Input: part model. Units: mm. Frame: model coordinates. A direction names the side the tool comes from. Coordinates: 2 decimals unless noted, no trailing zeros. Use a Markdown table: item, result. Add a question column.
Autodesk Inventor part; units mm, degrees
ref_plane "YZ Plane" through (0, 0, 0) normal (1, 0, 0) x (0, 1, 0)
ref_plane "XZ Plane" through (0, 0, 0) normal (0, 1, 0) x (-1, 0, 0)
ref_plane "XY Plane" through (0, 0, 0) normal (0, 0, 1) x (1, 0, 0)
sketch "Sketch1" plane through (0, 0, 0) normal (0, 1, 0) x (-1, 0, 0)
  line L0 (0, 0) -> (-40, 0)
  line L1 (-40, 0) -> (-40, -50)
  line L2 (-40, -50) -> (0, -50)
  line L3 (0, -50) -> (0, 0)
  dimension "d0" = 40
  dimension "d1" = 50
extrude "Extrusion1" add sketch "Sketch1" along normal blind 100
move faces "Move1" translate (0, 0, -13) faces at (13.3333, 33.3333, 0)
sketch "Sketch2" plane through (0, 0, -13) normal (0, 0, 1) x (1, 0, 0)
  line L0 (0, 0) -> (40, 0)
  line L1 (40, 0) -> (40, 100)
  line L2 (0, 100) -> (40, 100)
  line L3 (0, 0) -> (0, 100)
  line L4 (39, 99) -> (39, 1)
  line L5 (39, 1) -> (1, 1)
  line L6 (1, 1) -> (1, 99)
  line L7 (1, 99) -> (39, 99)
  dimension "d7" = 1
extrude "Extrusion2" add sketch "Sketch2" along normal blind 2 contours L4 L5 L6 L7
sketch "Sketch3" plane through (0, 0, -11) normal (0, 0, 1) x (1, 0, 0)
  line L0 (0, 100) -> (40, 100)
  line L1 (0, 0) -> (0, 100)
  line L2 (40, 0) -> (40, 100)
  line L3 (0, 0) -> (40, 0)
extrude "Extrusion3" add sketch "Sketch3" along normal blind 12
move faces "Move2" translate (3, 0, 0) faces at (40, 66.6667, -37.6667) (39, 33.6667, -12.3333) (40, 33.3333, -7)
move faces "Move3" translate (0, -3, 0) faces at (28.6667, 100, -25.3333) (14.6667, 99, -11.6667) (14.3333, 100, -3)
sketch "Sketch4" plane through (0, 0, 1) normal (0, 0, 1) x (1, 0, 0)
  line L0 (0, 97) -> (0, 0)
  line L1 (0, 0) -> (43, 0)
  line L2 (43, 0) -> (43, 97)
  line L3 (43, 97) -> (0, 97)
  line L4 (1, 96) -> (1, 1)
  line L5 (1, 1) -> (42, 1)
  line L6 (42, 1) -> (42, 96)
  line L7 (42, 96) -> (1, 96)
  line L8 (1, 96) -> (42, 96)
  line L9 (1, 96) -> (11, 96)
  line L10 (11, 96) -> (11, 86)
  line L11 (11, 86) -> (1, 86)
  line L12 (1, 86) -> (1, 96)
  line L13 (42, 96) -> (32, 96)
  line L14 (32, 96) -> (32, 86)
  line L15 (32, 86) -> (42, 86)
  line L16 (42, 86) -> (42, 96)
  dimension "d18" = 1
  dimension "d19" = 10
  dimension "d20" = 10
  dimension "d21" = 10
  dimension "d22" = 10
extrude "Extrusion4" cut sketch "Sketch4" against normal blind 0.5 contours L7 L10 L11 L4 | L7 L6 L15 L14
ref_plane "Work Plane1" through (0, 48.5, 0) normal (0, -1, 0) x (1, 0, 0)
equation "\"d22\" = d20"
properties part number "1.4AH SLAB"
1) Contact query for flat-ended pins moving along their axis: P1, Ø3, axis at x = 35, y = 90, coming from the +Z side; P2, Ø8, axis at x = 7.5, y = 90, coming from the +Z side; P3, Ø0.6, axis at x = 30.5, z = -12, coming from the +Y side; P4, Ø0.6, axis at x = 20, z = -11.5, coming from the -Y side. Output: stop coordinate, or through.
2) Material intervals for L1, parallel to Y at x = 34.5, z = -12, sorted ascending.
3) Pull-direction query (Z, two-part tool) for faces 1 (the flat face through (6, 91, 0.5)), 2 (the flat face through (22, 0, -31)), 3 (the flat face through (1, 48, -12)); classes: pulls with the +Z half, pulls with the -Z half, needs draft (parallel to the pull), parting line crosses it, or undercut.
4) Reachability of faces 4 (the flat face through (21, 96, -12)), 5 (the flat face through (42, 49, -12)), 6 (the flat face through (22, 1, -12)) from +Z, -Z, +X, -X, +Y, -Y: full face, straight path, thin tool, end or side. Return the list, or none.
Computed:
| question | item | result |
|---|---|---|
| 1 | P1 | stops at z = 0.5 |
| 1 | P2 | stops at z = 1 |
| 1 | P3 | stops at y = 96 |
| 1 | P4 | stops at y = 1 |
| 2 | L1 | y = 1 to 96 |
| 3 | face 1 | pulls with the +Z half |
| 3 | face 2 | needs draft |
| 3 | face 3 | undercut |
| 4 | face 4 | +X, -X, +Y |
| 4 | face 5 | +X, +Y, -Y |
| 4 | face 6 | +X, -X, -Y |
